Geometry: final body of the model. Coordinates: model frame, mm. Face numbers are marked on the shaded views. A direction names the side the tool comes from. Round coordinates to 2 decimals unless told otherwise and drop trailing zeros. Order: outer loops, then holes, each group sorted by start corner. A loop starts at its lowest first (then second) coordinate and runs counter-clockwise, first axis right, second up. Notation, with made-up numbers: (-27.75, 43.5) -> (14.25, 43.5) arc R19 cw to (14.25, 55.5) -> close; hole circle Ø4 at (36.5, 66.5). An arc over 180 degrees is marked (long way). Put each result on its own line as item: value.
```python
from build123d import *

# Parameters (mm, degrees)
SKETCH1_W                       = 3
SKETCH1_H                       = 8
BOSS_EXTRUDE1_DEPTH             = 8
SKETCH2_W                       = 15
SKETCH2_H                       = 8
BOSS_EXTRUDE2_DEPTH             = 3
SKETCH3_R                       = 2.575
CUT_EXTRUDE1_DEPTH              = 3
FILLET1_R                       = 4
SKETCH4_W                       = 4
SKETCH4_H                       = 1.75
BOSS_EXTRUDE3_DEPTH             = 10
BOSS_EXTRUDE3_DIRECTION_2_REACH = 21.164
SKETCH5_R                       = 1.05
CUT_EXTRUDE2_DEPTH              = 3
FILLET2_R                       = 2
FILLET3_R                       = 1.25
FILLET1_OF_MIRROR1_R            = 4
FILLET2_OF_MIRROR1_R            = 2
FILLET3_OF_MIRROR1_R            = 1.25


with BuildPart() as part:
    # Sketch1 → Boss-Extrude1 (new body)
    with BuildSketch(Plane(origin=(0, 0, 0), x_dir=(1, 0, 0), z_dir=(0, 1, 0))):
        Rectangle(SKETCH1_W, SKETCH1_H)
    boss_extrude1 = extrude(amount=BOSS_EXTRUDE1_DEPTH)

    # Sketch2 → Boss-Extrude2 (add)
    with BuildSketch(Plane(origin=(0, 8, 0), x_dir=(1, 0, 0), z_dir=(0, 1, 0))):
        with Locations((-6, 0)):
            Rectangle(SKETCH2_W, SKETCH2_H)
    boss_extrude2 = extrude(amount=BOSS_EXTRUDE2_DEPTH)

    # Sketch3 → Cut-Extrude1 (cut)
    with BuildSketch(Plane(origin=(0, 11, 0), x_dir=(1, 0, 0), z_dir=(0, 1, 0))):
        with Locations(Location((-9.25, 0, 0), (0, 0, 270))):
            Circle(SKETCH3_R)
    cut_extrude1 = extrude(amount=-CUT_EXTRUDE1_DEPTH, mode=Mode.SUBTRACT)

    # Fillet1
    fillet1_edges = [part.edges().sort_by_distance(p)[0] for p in [
        (-13.5, 9.5, 4),
        (-13.5, 9.5, -4),
    ]]
    fillet(fillet1_edges, radius=FILLET1_R - 0.0001)  # a hair under: the kernel refuses the full size

    # Sketch4 → Boss-Extrude3 (add)
    with BuildSketch(Plane.XY.offset(4)):
        with Locations((-9.25, 10.125)):
            Rectangle(SKETCH4_W, SKETCH4_H)
    boss_extrude3 = extrude(amount=BOSS_EXTRUDE3_DEPTH)

    # Sketch4 → Boss-Extrude3 direction 2 (add, up to next)
    with BuildSketch(Plane.XY.offset(4), mode=Mode.PRIVATE) as boss_extrude3_direction_2_sk1:
        with Locations((-9.25, 10.125)):
            Rectangle(SKETCH4_W, SKETCH4_H)
    boss_extrude3_direction_2_tool1 = extrude(boss_extrude3_direction_2_sk1.sketch, amount=-BOSS_EXTRUDE3_DIRECTION_2_REACH, mode=Mode.PRIVATE) - part.part
    boss_extrude3_direction_2 = boss_extrude3_direction_2_tool1.solids().sort_by_distance((-9.25, 10.125, 4))[0]
    add(boss_extrude3_direction_2)

    # Sketch5 → Cut-Extrude2 (cut)
    with BuildSketch(Plane(origin=(0, 11, 0), x_dir=(1, 0, 0), z_dir=(0, 1, 0))):
        with Locations(Location((-9.25, -12, 0), (0, 0, 270))):
            Circle(SKETCH5_R)
    cut_extrude2 = extrude(amount=-CUT_EXTRUDE2_DEPTH, mode=Mode.SUBTRACT)

    # Fillet2
    fillet2_edges = [part.edges().sort_by_distance(p)[0] for p in [
        (-11.25, 10.125, 14),
        (-7.25, 10.125, 14),
    ]]
    fillet(fillet2_edges, radius=FILLET2_R - 0.0001)  # a hair under: the kernel refuses the full size

    # Fillet3
    fillet3_edges = [part.edges().sort_by_distance(p)[0] for p in [
        (-8.37505, 9.25, 4),
        (-10.397962835, 9.25, 3.897925335),
    ]]
    fillet(fillet3_edges, radius=FILLET3_R - 0.0001)  # a hair under: the kernel refuses the full size

    # Mirror1: Boss-Extrude1, Boss-Extrude2, Cut-Extrude1, Boss-Extrude3, Boss-Extrude3 direction 2, Cut-Extrude2 across plane
    add(boss_extrude1.mirror(Plane.ZX))
    add(boss_extrude2.mirror(Plane.ZX))
    add(cut_extrude1.mirror(Plane.ZX), mode=Mode.SUBTRACT)
    add(boss_extrude3.mirror(Plane.ZX))
    add(boss_extrude3_direction_2.mirror(Plane.ZX))
    add(cut_extrude2.mirror(Plane.ZX), mode=Mode.SUBTRACT)

    # Fillet1 of Mirror1
    fillet1_of_mirror1_edges = [part.edges().sort_by_distance(p)[0] for p in [
        (-13.5, -9.5, 4),
        (-13.5, -9.5, -4),
    ]]
    fillet(fillet1_of_mirror1_edges, radius=FILLET1_OF_MIRROR1_R - 0.0001)  # a hair under: the kernel refuses the full size

    # Fillet2 of Mirror1
    fillet2_of_mirror1_edges = [part.edges().sort_by_distance(p)[0] for p in [
        (-11.25, -10.125, 14),
        (-7.25, -10.125, 14),
    ]]
    fillet(fillet2_of_mirror1_edges, radius=FILLET2_OF_MIRROR1_R - 0.0001)  # a hair under: the kernel refuses the full size

    # Fillet3 of Mirror1
    fillet3_of_mirror1_edges = [part.edges().sort_by_distance(p)[0] for p in [
        (-8.37505, -9.25, 4),
        (-10.397962835, -9.25, 3.897925335),
    ]]
    fillet(fillet3_of_mirror1_edges, radius=FILLET3_OF_MIRROR1_R - 0.0001)  # a hair under: the kernel refuses the full size


solid = part.part
```
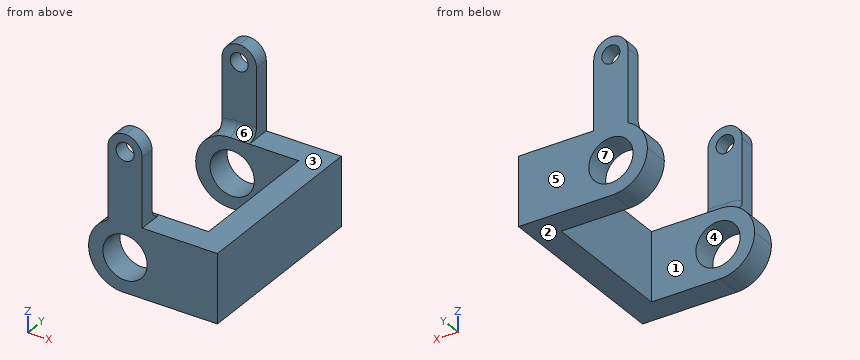
1. Set-up query: the marked faces 1, 2 and 3. Return all of +Z, -Z, +X, -X, +Y, -Y with unobstructed straight access to the full face (end or side cutting, diameter ignored); none if empty.
Ans:
face 1: +Z, -Z, -X
face 2: -Z, +X, -X, +Y, -Y
face 3: +Z, +X, +Y, -Y
2. Cut plane C-C on z = 12.75. Return loops of the section in (x, y).
Ans:
outline: (-11.1, -11) -> (-9.98, -11) -> (-9.98, -9.25) -> (-11.1, -9.25) -> close; (-11.1, 9.25) -> (-9.98, 9.25) -> (-9.98, 11) -> (-11.1, 11) -> close; (-8.52, -11) -> (-7.4, -11) -> (-7.4, -9.25) -> (-8.52, -9.25) -> close; (-8.52, 9.25) -> (-7.4, 9.25) -> (-7.4, 11) -> (-8.52, 11) -> close
3. Material intervals for probe 1 along X at (y, z) = (9.8, 0) (3 decimals); probe 2 along X at (y, z) = (-10.25, 12); probe 3 along Y at (x, z) = (-3.5, -2.5), sorted ascending.
Ans:
probe 1: -13.5 to -11.825, -6.675 to 1.5
probe 2: -11.25 to -10.3, -8.2 to -7.25
probe 3: -11 to -8, 8 to 11
4. Contact query for flat-ended pins moving along their axis: P1, Ø1.5, axis at y = 9.5, z = 6, coming from the -X side; P2, Ø4, axis at x = -9.25, z = 0, coming from the +Y side; P3, Ø5, axis at x = -9.5, z = -0.5, coming from the -Y side; P4, Ø5, axis at x = -2, y = 4.5, coming from the +Z side. Output: stop coordinate, or through.
Ans:
P1: x = -11.25
P2: through
P3: y = -11
P4: z = 4
5. Cut plane D-D on y = 1.75. Return loops of the section in (x, z), and give its area (3 significant figures).
Ans:
outline: (-1.5, -4) -> (1.5, -4) -> (1.5, 4) -> (-1.5, 4) -> close
area: 24.0 mm²
6. Draft query along Z for the marked faces 4, 5, 6 and 7. Return one class per face: +Z half, -Z half, draft (parallel to the pull), parting line (faces both ways), or undercut.
Ans:
face 4: undercut
face 5: draft
face 6: +Z half
face 7: undercut
7. Cut plane B-B on z = -1.25. Return loops of the section in (x, y), and give its area (3 significant figures).
Ans:
outline: (-13.3, -11) -> (-11.5, -11) -> (-11.5, -8) -> (-13.3, -8) -> close; (-13.3, 8) -> (-11.5, 8) -> (-11.5, 11) -> (-13.3, 11) -> close; (-7, -11) -> (1.5, -11) -> (1.5, 11) -> (-7, 11) -> (-7, 8) -> (-1.5, 8) -> (-1.5, -8) -> (-7, -8) -> close
area: 110 mm²
8. Cut plane A-A on x = -6. Return loops of the section in (y, z).
Ans:
outline: (-11, -4) -> (-8, -4) -> (-8, 4) -> (-11, 4) -> close; (8, -4) -> (11, -4) -> (11, 4) -> (8, 4) -> close
